Model file for the job. Use its own axes, mm. Face numbers are marked on the shaded views. Give positions to 0.01 mm unless a question says otherwise; leave off trailing zeros. Loops run counter-clockwise (first coordinate to the right, second up) from the corner with the lowest first, then second, coordinate; pieces in that order, holes last. Notation, with made-up numbers: (-37.75, -26) -> (-27.75, -26) arc R24 cw to (-27.75, 2) -> close; hole circle Ø7 at (56.5, 28). An arc over 180 degrees is marked (long way). Use CSV: the item, a comma, the result in double quotes. Start each with the question number.
(1) Pull direction Y, two halves, no side cores. Call the marked faces 1, 2 and 3: pulls with the +Y half, pulls with the -Y half, needs draft (parallel to the pull), parting line crosses it, or undercut.
(2) Cut at A-A on z = 2.75. Write the cut outline in (x, y), then the cut area to 3 significant figures.
(3) Cut at B-B on x = 0. Write the cut outline in (y, z), then the cut area to 3 significant figures.
(4) Cut at D-D on x = -12. Write the cut outline in (y, z), then the cut area to 3 significant figures.
(5) Cut at C-C on y = 0. Write the cut outline in (x, z).
(6) Drill centre lines: probe 1 along Z at (x, y) = (-8, -4); probe 2 along Y at (x, z) = (2.5, 6); probe 3 along X at (y, z) = (0.5, 7.5). Where is each one in solid material? Low to high.
(7) Flat gauge pins, fed straight in: pin 1 (3.5 mm diameter, centred on y = -0.5, z = 5, fed in from +X); pin 2 (5 mm diameter, centred on x = 1, z = 4, fed in from -Y); pin 3 (5 mm diameter, centred on x = -16, y = -3, fed in from -Z); pin 4 (2 mm diameter, centred on y = -14, z = 2, fed in from -X). Where does each tip first touch, or does it go through?
Autodesk Inventor part; units mm, degrees
ref_plane "YZ Plane" through (0, 0, 0) normal (1, 0, 0) x (0, 1, 0)
ref_plane "XZ Plane" through (0, 0, 0) normal (0, 1, 0) x (-1, 0, 0)
ref_plane "XY Plane" through (0, 0, 0) normal (0, 0, 1) x (1, 0, 0)
sketch "Sketch1" plane through (0, 0, 0) normal (0, 0, 1) x (1, 0, 0)
  circle A0 centre (0, 0) radius 20
  dimension "d0" = 40
extrude "Extrusion1" add sketch "Sketch1" along normal blind 2
sketch "Sketch2" plane through (0, 0, 2) normal (0, 0, 1) x (1, 0, 0)
  circle A0 centre (0, 0) radius 4
  dimension "d3" = 8
extrude "Extrusion2" add sketch "Sketch2" along normal blind 7
sketch "Sketch3" plane through (0, 0, 9) normal (0, 0, 1) x (1, 0, 0)
  line L0 (-3, 1.5) -> (3, 1.5)
  line L1 (3, 1.5) -> (3, -1.5)
  line L2 (3, -1.5) -> (-3, -1.5)
  line L3 (-3, -1.5) -> (-3, 1.5)
  point P0 (0, 0)
  dimension "d6" = 6
  dimension "d7" = 3
  dimension "d8" = 1.5
  dimension "d9" = 3
  dimension "d10" = 3
extrude "Extrusion3" cut sketch "Sketch3" against normal blind 7
properties part number "baser"
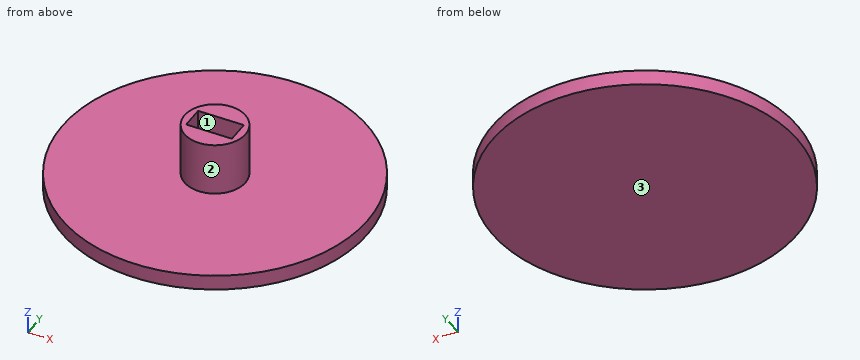
Check result:
1,face 1,"undercut"
1,face 2,"parting line crosses it"
1,face 3,"needs draft"
2,outline,"circle Ø8 at (0, 0); hole (-3, -1.5) -> (3, -1.5) -> (3, 1.5) -> (-3, 1.5) -> close"
2,area,"32.3 mm²"
3,outline,"(-20, 0) -> (20, 0) -> (20, 2) -> (4, 2) -> (4, 9) -> (1.5, 9) -> (1.5, 2) -> (-1.5, 2) -> (-1.5, 9) -> (-4, 9) -> (-4, 2) -> (-20, 2) -> close"
3,area,"115 mm²"
4,outline,"(-16, 0) -> (16, 0) -> (16, 2) -> (-16, 2) -> close"
4,area,"64.0 mm²"
5,outline,"(-20, 0) -> (20, 0) -> (20, 2) -> (4, 2) -> (4, 9) -> (3, 9) -> (3, 2) -> (-3, 2) -> (-3, 9) -> (-4, 9) -> (-4, 2) -> (-20, 2) -> close"
6,probe 1,"0 to 2"
6,probe 2,"-3.12 to -1.5, 1.5 to 3.12"
6,probe 3,"-3.97 to -3, 3 to 3.97"
7,pin 1,"x = 4"
7,pin 2,"y = -20"
7,pin 3,"z = 0"
7,pin 4,"x = -15.2"
